Geometry: see drawing. Coordinates: mm, zero at the bounding-box minimum. A direction names the side the tool comes from. Give positions to 0.01 mm unless a question says otherwise; leave off trailing zeros. Order: outer loops, then holes, each group sorted by start corner. A loop starts at its lowest first (then second) coordinate and runs counter-clockwise, first axis right, second up. Notation, with made-up numbers: M -16,54 L 15,54 A15 ccw 15,71 Z; hole C -5.75,89 d7. An arc over 180 degrees is marked long. Use a Markdown table: item, result.
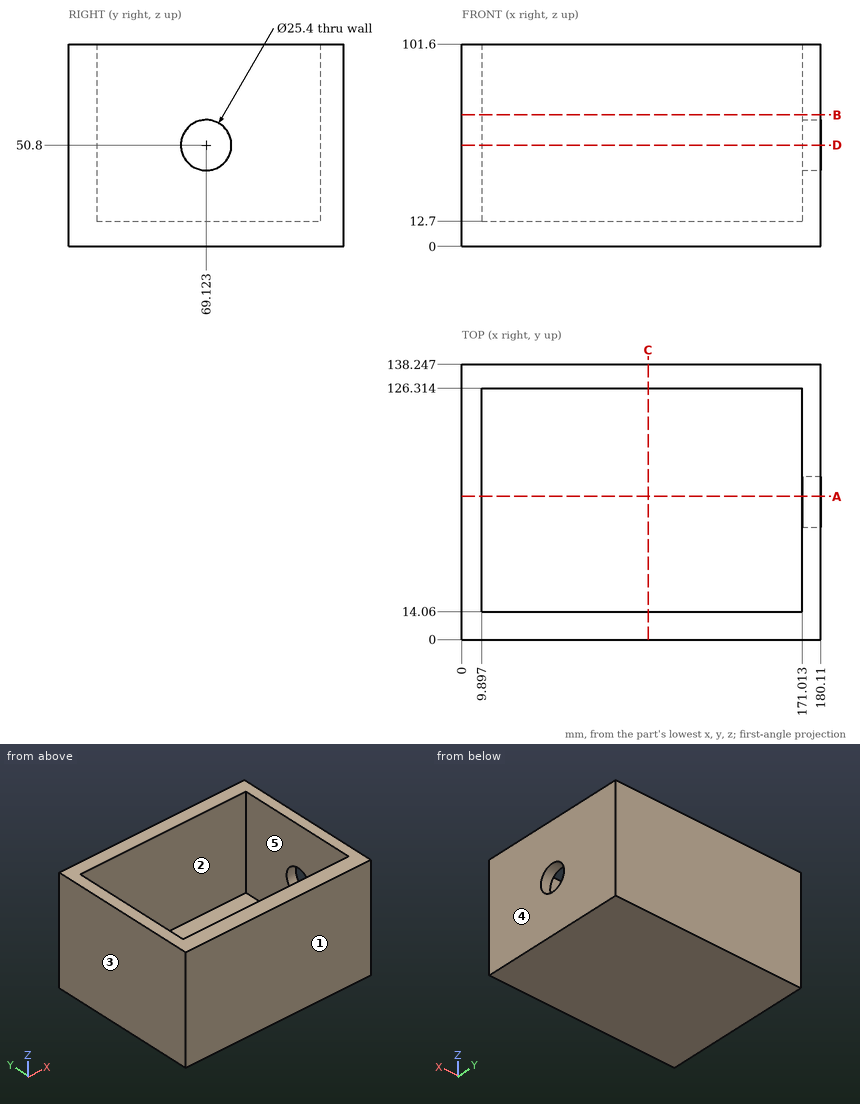
1) Mould query, pull axis Y, two halves, no side actions, for the marked faces 1, 2 and 3. Classes: released by +Y, released by -Y, zero draft, split by the parting line, or undercut.
Response values:
| item | result |
|---|---|
| face 1 | released by -Y |
| face 2 | undercut |
| face 3 | zero draft |
2) Cut plane B-B on z = 66. Return loops of the section in (x, y).
Response values:
| item | result |
|---|---|
| outline | M 0,0 L 180.11,0 L 180.11,138.25 L 0,138.25 Z; hole M 9.9,14.06 L 171.01,14.06 L 171.01,126.31 L 9.9,126.31 Z |
3) Cut plane D-D on z = 50.8. Return loops of the section in (x, y), and give its area (3 significant figures).
Response values:
| item | result |
|---|---|
| outline | M 0,0 L 180.11,0 L 180.11,56.42 L 171.01,56.42 L 171.01,14.06 L 9.9,14.06 L 9.9,126.31 L 171.01,126.31 L 171.01,81.82 L 180.11,81.82 L 180.11,138.25 L 0,138.25 Z |
| area | 6,580 mm² |
4) Reachability of the marked faces 4 and 5 from +Z, -Z, +X, -X, +Y, -Y: full face, straight path, thin tool, end or side. Return the list, or none.
Response values:
| item | result |
|---|---|
| face 4 | +Z, -Z, +X, +Y, -Y |
| face 5 | +Z |
5) Material intervals for line 1 (X direction, y = 116.5, z = 34); line 2 (Y direction, x = 65.5, z = 49.5); line 3 (Z direction, x = 54.5, y = 109), sorted ascending. Write a range as from..to.
Response values:
| item | result |
|---|---|
| line 1 | x = 0..9.9, 171.01..180.11 |
| line 2 | y = 0..14.06, 126.31..138.25 |
| line 3 | z = 0..12.7 |
6) First-contact query: pin 1 Ø23 at (y, z) = (69.12, 50.8) entering from +X; pin 2 Ø2 at (x, y) = (121.5, 121) entering from +Z. Flat tips, straight axial feed; report the tip coordinate or a pass-through.
Response values:
| item | result |
|---|---|
| pin 1 | stops at x = 9.9 |
| pin 2 | stops at z = 12.7 |
7) Cut plane C-C on x = 93.5. Return loops of the section in (y, z).
Response values:
| item | result |
|---|---|
| outline | M 0,0 L 138.25,0 L 138.25,101.6 L 126.31,101.6 L 126.31,12.7 L 14.06,12.7 L 14.06,101.6 L 0,101.6 Z |
8) Cut plane A-A on y = 72. Return loops of the section in (x, z).
Response values:
| item | result |
|---|---|
| outline | M 0,0 L 180.11,0 L 180.11,38.43 L 171.01,38.43 L 171.01,12.7 L 9.9,12.7 L 9.9,101.6 L 0,101.6 Z; M 171.01,63.17 L 180.11,63.17 L 180.11,101.6 L 171.01,101.6 Z |
